from build123d import *

# Parameters (mm, degrees)
SALIENTE_EXTRUIR1_DEPTH = 20
CORTAR_EXTRUIR1_DEPTH   = 5.3


with BuildPart() as part:
    # Croquis3 → Saliente-Extruir1 (new body)
    with BuildSketch(Plane.XY):
        with BuildLine():
            Line((-51.952746953, -11.691023914), (-51.874375972, -12.286308051))
            Line((-51.874375972, -12.286308051), (-51.644609193, -12.841022845))
            Line((-51.644609193, -12.841022845), (-51.279094792, -13.317369615))
            Line((-51.279094792, -13.317369615), (-50.802748021, -13.68288106))
            Line((-50.802748021, -13.68288106), (-50.24803027, -13.912653752))
            Line((-50.24803027, -13.912653752), (-49.65250662, -13.99148306))
            Line((-49.65250662, -13.99148306), (-48.634298914, -14.325284182))
            Line((-48.634298914, -14.325284182), (-47.63492106, -14.711825449))
            Line((-47.63492106, -14.711825449), (-46.657105279, -15.15005123))
            Line((-46.657105279, -15.15005123), (-45.70351874, -15.638763962))
            Line((-45.70351874, -15.638763962), (-44.776769471, -16.17663006))
            Line((-44.776769471, -16.17663006), (-43.879382708, -16.762176963))
            Line((-43.879382708, -16.762176963), (-43.013812718, -17.393807919))
            Line((-43.013812718, -17.393807919), (-42.182430974, -18.069799027))
            Line((-42.182430974, -18.069799027), (-41.387496586, -18.788302193))
            Line((-41.387496586, -18.788302193), (-40.631179954, -19.547354003))
            Line((-40.631179954, -19.547354003), (-39.91556277, -20.344881636))
            Line((-39.91556277, -20.344881636), (-39.24257888, -21.178708777))
            Line((-39.24257888, -21.178708777), (-41.33719888, -25.732864397))
            Line((-41.33719888, -25.732864397), (-42.055027862, -30.693958319))
            Line((-42.055027862, -30.693958319), (-40.034201485, -30.693958319))
            Line((-40.034201485, -30.693958319), (-39.399249875, -26.305668328))
            Line((-39.399249875, -26.305668328), (-37.546478747, -22.277332194))
            Line((-37.546478747, -22.277332194), (-34.627863462, -18.93937864))
            Line((-34.627863462, -18.93937864), (-30.882804538, -16.565607853))
            Line((-30.882804538, -16.565607853), (-26.81051779, -15.405439974))
            Line((-26.81051779, -15.405439974), (-26.618493511, -15.3507305))
            Line((-26.618493511, -15.3507305), (-22.195772803, -15.394292275))
            Line((-22.195772803, -15.394292275), (-4.431072692, -19.454792623))
            Line((-4.431072692, -19.454792623), (-4.431072692, -41.693958205))
            Line((-4.431072692, -41.693958205), (-1.951072692, -41.693958205))
            Line((-1.951072692, -41.693958205), (-1.951072692, -10.693958394))
            Line((-1.951072692, -10.693958394), (-14.311475216, -10.693958394))
            Line((-14.311475216, -10.693958394), (-14.311475216, -4.693956642))
            Line((-14.311475216, -4.693956642), (-24.311475179, -4.693956642))
            Line((-24.311475179, -4.693956642), (-24.311475179, -7.693958997))
            Line((-24.311475179, -7.693958997), (-18.31147047, -7.693958997))
            ThreePointArc((-18.31147047, -7.693958997), (-17.604362437, -7.986851509), (-17.311465743, -8.69395781))
            Line((-17.311465743, -8.69395781), (-17.311465743, -11.993957443))
            Line((-17.311465743, -11.993957443), (-31.952510471, -11.993957443))
            Line((-31.952510471, -11.993957443), (-31.952510471, -9.293958281))
            Line((-31.952510471, -9.293958281), (-36.952504539, -9.293958281))
            Line((-36.952504539, -9.293958281), (-36.952504539, -11.293958865))
            Line((-36.952504539, -11.293958865), (-49.952506856, -11.293958865))
            Line((-49.952506856, -11.293958865), (-49.952506856, -1.693957245))
            Line((-49.952506856, -1.693957245), (-51.951481378, -1.69383601))
            Line((-51.951481378, -1.69383601), (-51.952746953, -11.691023914))
        make_face()
    extrude(amount=SALIENTE_EXTRUIR1_DEPTH)

    # Croquis4 → Cortar-Extruir1 (cut)
    with BuildSketch(Plane(origin=(0, 0, 0), x_dir=(-1, 0, 0), z_dir=(0, 0, -1))):
        Polygon((49.952506856, -11.293958865), (49.950268445, -13.952068406), (50.24803027, -13.912653752), (50.802748021, -13.68288106), (51.279094792, -13.317369615), (51.644609193, -12.841022845), (51.874375972, -12.286308051), (51.952746953, -11.691023914), (51.951481378, -1.69383601), (49.952506856, -1.693957245), align=None)
    extrude(amount=-CORTAR_EXTRUIR1_DEPTH, mode=Mode.SUBTRACT)


solid = part.part
Check sheet for the modelled part. Datum: model origin and axes. Units: mm. A direction names the side the tool comes from. Coordinates: 2 decimals unless noted, no trailing zeros. Loops run counter-clockwise (first coordinate to the right, second up) from the corner with the lowest first, then second, coordinate; pieces in that order, holes last. Notation, with made-up numbers: (-40, 27.5) -> (-5, 27.5) arc R18 ccw to (-5, 47.5) -> close; hole circle Ø4 at (74.5, -39). An arc over 180 degrees is marked (long way). Answer in a Markdown table with one row per item.
1. Sectioned sample at A-A, the plane x = -23. Record the boundary of the cut face in (y, z), then the cut area to 3 significant figures.
Check values:
| item | result |
|---|---|
| outline | (-15.39, 0) -> (-11.99, 0) -> (-11.99, 20) -> (-15.39, 20) -> close; (-7.69, 0) -> (-4.69, 0) -> (-4.69, 20) -> (-7.69, 20) -> close |
| area | 128 mm2 |
2. Material ranges on line 1 along X through (y, z) = (-11.5, 14); line 2 along X through (y, z) = (-9, 15.5); line 3 along Y through (x, z) = (-24, 6), recorded low to high. Write a range as [from, to].
Check values:
| item | result |
|---|---|
| line 1 | x = [-51.95, -31.95], [-17.31, -1.95] |
| line 2 | x = [-51.95, -49.95], [-17.31, -14.31] |
| line 3 | y = [-15.38, -11.99], [-7.69, -4.69] |
3. Release check for a two-part mould opening along Y. For faces 1 (the face through (-3, -41.694, 10)), 2 (the face through (-36.953, -10, 10)), 3 (the face through (-25, -11.994, 10)) record: released by +Y, released by -Y, zero draft, split by the parting line, or undercut.
Check values:
| item | result |
|---|---|
| face 1 | released by -Y |
| face 2 | zero draft |
| face 3 | undercut |
4. Sectioned sample at B-B, the plane y = -29. Record the boundary of the cut face in (x, z).
Check values:
| item | result |
|---|---|
| outline | (-41.81, 0) -> (-39.79, 0) -> (-39.79, 20) -> (-41.81, 20) -> close; (-4.43, 0) -> (-1.95, 0) -> (-1.95, 20) -> (-4.43, 20) -> close |
5. Go/stop test with flat-tipped pins: pin 1 (1.6 mm diameter, centred on x = -51, y = -7.5, fed in from -Z); pin 2 (5 mm diameter, centred on x = -22.5, z = 9, fed in from -Y); pin 3 (2 mm diameter, centred on y = -19, z = 14.5, fed in from -X). Record where each tip stops, or that it passes through.
Check values:
| item | result |
|---|---|
| pin 1 | stops at z = 5.3 |
| pin 2 | stops at y = -15.9 |
| pin 3 | stops at x = -42.27 |
6. Sectioned sample at D-D, the plane x = -9. Record the boundary of the cut face in (y, z), then the cut area to 3 significant figures.
Check values:
| item | result |
|---|---|
| outline | (-18.41, 0) -> (-10.69, 0) -> (-10.69, 20) -> (-18.41, 20) -> close |
| area | 154 mm2 |
7. Access from +Z, -Z, +X, -X, +Y, -Y to the whole of each face (thin tool, end or side, straight path). Record for faces 4 (the face through (-31.953, -11, 10)), 5 (the face through (-14.311, -8, 10)), 6 (the face through (-49.151, -14.156, 9.86)), 7 (the face through (-21, -7.694, 10)), 8 (the face through (-36.108, -20.632, 9.86)).
Check values:
| item | result |
|---|---|
| face 4 | +Z, -Z, +Y |
| face 5 | +Z, -Z, +X, +Y |
| face 6 | +Z, -Z, -X, -Y |
| face 7 | +Z, -Z |
| face 8 | +Z, -Z, -Y |
8. Sectioned sample at C-C, the plane y = -36. Record the boundary of the cut face in (x, z), then the cut area to 3 significant figures.
Check values:
| item | result |
|---|---|
| outline | (-4.43, 0) -> (-1.95, 0) -> (-1.95, 20) -> (-4.43, 20) -> close |
| area | 49.6 mm2 |
